Source: CAD feature listing. Evaluate the final solid. Frame: model axes, mm. Coordinates: 2 decimals unless noted, no trailing zeros. Write each loop counter-clockwise with the first axis right and the second up, starting at its lowest first coordinate (ties: lowest second). Pieces come first, ordered by that corner, then holes. Notation, with made-up numbers: (-22.5, 66) -> (-8.5, 66) arc R19 cw to (-8.5, 102) -> close; hole circle Ø7 at (69, 76.25). An arc over 180 degrees is marked (long way). One line per item, written item: value. Start each with the question number.
1. Section query A-A, the plane y = -37.5. Output: boundary loops of the cut face in (x, z), and give its area (3 significant figures).
2. First-contact query: P1, Ø2.5, axis at x = 18.8, y = 62.5, coming from the -Z side; P2, Ø3.5, axis at x = 18.85, y = 37.5, coming from the -Z side. Flat tips, straight axial feed; report the tip coordinate or a pass-through.
3. Line query: line 1 (Y direction, x = -35.5, z = 4.5). Output: solid intervals per line, ascending.
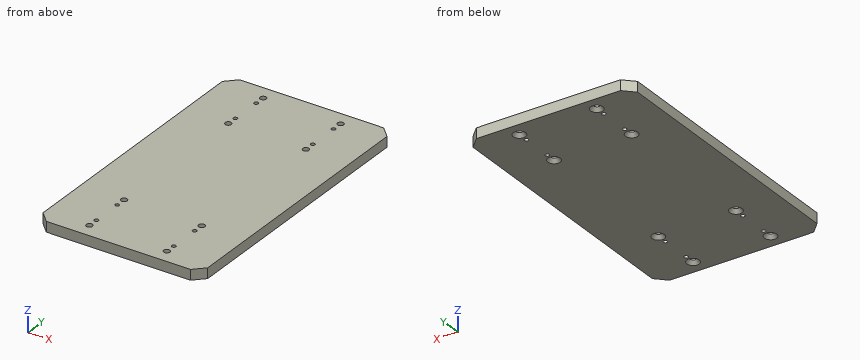
from build123d import *

# Parameters (mm, degrees)
SKETCH1_W                = 80
SKETCH1_H                = 139
BOSS_EXTRUDE1_DEPTH      = 5
F_3_0_3_DIAMETER_HOLE1_D = 3
F_2_0_2_DIAMETER_HOLE1_D = 2
CHAMFER1_SIZE            = 1.5
CHAMFER1_SIZE2           = 1.787630389
CHAMFER2_SIZE            = 5


with BuildPart() as part:
    # Sketch1 → Boss-Extrude1 (new body)
    with BuildSketch(Plane.XY.offset(5)):
        Rectangle(SKETCH1_W, SKETCH1_H)
    extrude(amount=-BOSS_EXTRUDE1_DEPTH)

    # Ø3.0 (3) Diameter Hole1 (through all)
    with Locations(Plane(origin=(0, 0, 0), x_dir=(-1, 0, 0), z_dir=(0, 0, -1))):
        with Locations((-18.8, 62.5), (18.8, -62.5), (-18.84545318, -37.5), (18.84545318, -37.5), (18.8, 62.5), (-18.84545318, 37.5), (18.84545318, 37.5), (-18.8, -62.5)):
            Hole(F_3_0_3_DIAMETER_HOLE1_D / 2)

    # Ø2.0 (2) Diameter Hole1 (through all)
    with Locations(Plane(origin=(0, 0, 0), x_dir=(-1, 0, 0), z_dir=(0, 0, -1))):
        with Locations((-18.8, 42.5), (-18.8, 57.5), (18.8, 42.5), (-18.8, -57.5), (-18.8, -42.5), (18.8, -57.5), (18.8, -42.5), (18.8, 57.5)):
            Hole(F_2_0_2_DIAMETER_HOLE1_D / 2)

    # Chamfer1
    chamfer1_edges = [part.edges().sort_by_distance(p)[0] for p in [
        (17.3, -62.5, 0),
        (-20.34545318, 37.5, 0),
        (17.34545318, 37.5, 0),
        (-20.3, 62.5, 0),
        (-20.34545318, -37.5, 0),
        (17.34545318, -37.5, 0),
        (-20.3, -62.5, 0),
        (17.3, 62.5, 0),
    ]]
    chamfer1_side = [part.faces().sort_by_distance(p)[0] for p in [
        (0, 0, 0),
    ]]
    chamfer(chamfer1_edges, length=CHAMFER1_SIZE, length2=CHAMFER1_SIZE2, reference=chamfer1_side[0])

    # Chamfer2
    chamfer2_edges = [part.edges().sort_by_distance(p)[0] for p in [
        (-40, 69.5, 2.5),
        (40, 69.5, 2.5),
        (40, -69.5, 2.5),
        (-40, -69.5, 2.5),
    ]]
    chamfer(chamfer2_edges, length=CHAMFER2_SIZE)


solid = part.part
Computed values:
1. outline: (-40, 0) -> (-21.85, 0) -> (-20.35, 1.79) -> (-20.35, 5) -> (-40, 5) -> close; (-17.35, 1.79) -> (-15.85, 0) -> (15.85, 0) -> (17.35, 1.79) -> (17.35, 5) -> (-17.35, 5) -> close; (20.35, 1.79) -> (21.85, 0) -> (40, 0) -> (40, 5) -> (20.35, 5) -> close
1. area: 365 mm²
2. P1: passes through
2. P2: stops at z = 1.48
3. line 1: y = -69 to 69
